Job drawing, mm, ordinate dimensions from the low corner. One solid piece. A direction names the side the tool comes from. Give positions to 0.01 mm unless a question says otherwise; leave off trailing zeros. Order: outer loops, then holes, each group sorted by start corner. A loop starts at its lowest first (then second) coordinate and runs counter-clockwise, first axis right, second up. Notation, with made-up numbers: (67, -21) - (95, -21) arc R17 cw to (95, 3) - close; hole circle Ø7 at (-26.75, 48). An arc over 180 degrees is marked (long way). Write each question's results on one line, items separated by ' | '. Start each with the question number.
1) Cut at A-A on x = 5. List the corners of the cut face in (y, z), plus the area to 3 significant figures.
2) Cut at D-D on y = 38. List the corners of the cut face in (x, z), plus the area to 3 significant figures.
3) Drill centre lines: line 1 along X through (y, z) = (4, 5) (1 decimal); line 2 along Y through (x, z) = (35, 0.9); line 3 along Y through (x, z) = (11, 6). Where is each one in solid material? Low to high. Write a range as from..to.
4) Two-plate mould, pull along X, no slides. Class the marked faces 1, 2 and 3: +X half, -X half, draft (parallel to the pull), parting line (faces both ways), or undercut.
5) Drop flat-ended pins along their axis: pin 1 Ø2 at (x, z) = (59, 4) entering from -Y; pin 2 Ø1 at (y, z) = (19, 1.5) entering from +X; pin 3 Ø4.5 at (x, z) = (5, 4) entering from -Y; pin 4 Ø15 at (x, y) = (29, 14) entering from +Z. Give the stop position or say it passes through.
6) Cut at B-B on y = 24. List the corners of the cut face in (x, z), plus the area to 3 significant figures.
7) Tool access for the marked faces 4, 5, 6, 7 and 8: list every direction of +Z, -Z, +X, -X, +Y, -Y with a clear straight run to the whole face (end or side of a thin tool).
8) Cut at C-C on z = 4. State how many separate pieces and enclosed holes the cut face has, plus the area to 3 significant figures.
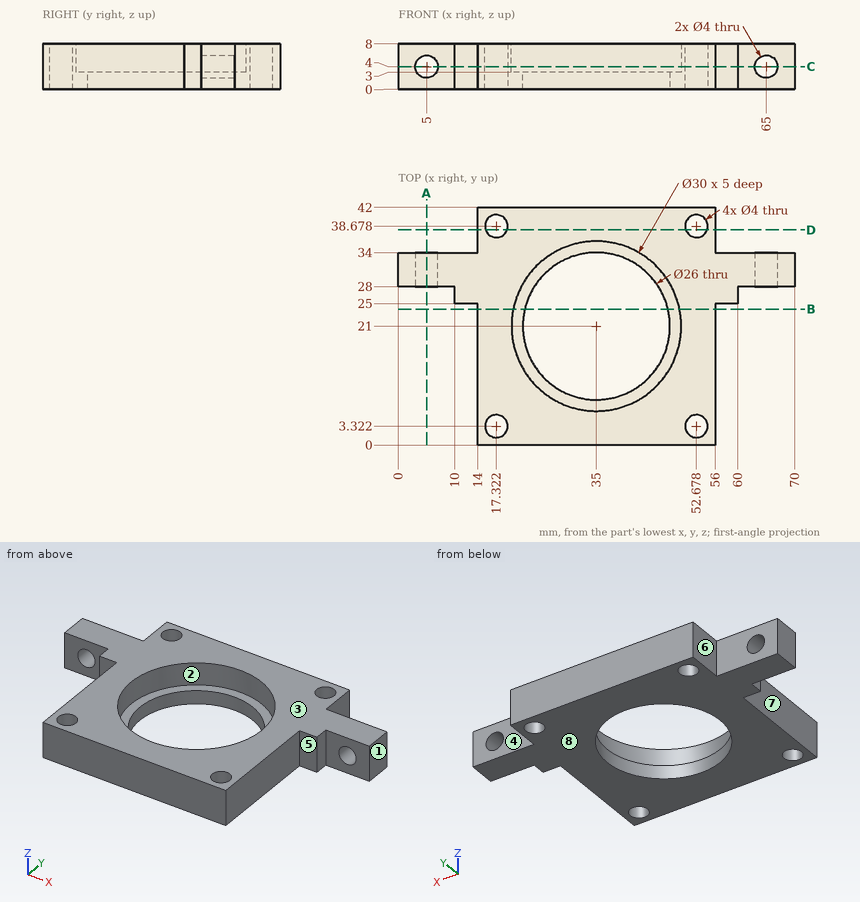
Results:
1) outline: (28, 0) - (34, 0) - (34, 2) - (28, 2) - close; (28, 6) - (34, 6) - (34, 8) - (28, 8) - close | area: 24.0 mm^2
2) outline: (14, 0) - (15.44, 0) - (15.44, 8) - (14, 8) - close; (19.2, 0) - (50.8, 0) - (50.8, 8) - (19.2, 8) - close; (54.56, 0) - (56, 0) - (56, 8) - (54.56, 8) - close | area: 276 mm^2
3) line 1: 14..15.4, 19.2..50.8, 54.6..56 | line 2: 0..8, 34..42 | line 3: 25..34
4) face 1: +X half | face 2: undercut | face 3: draft
5) pin 1: y = 25 | pin 2: x = 56 | pin 3: y = 28 | pin 4: z = 8
6) outline: (14, 0) - (22.35, 0) - (22.35, 3) - (20.3, 3) - (20.3, 8) - (14, 8) - close; (47.65, 0) - (56, 0) - (56, 8) - (49.7, 8) - (49.7, 3) - (47.65, 3) - close | area: 113 mm^2
7) face 4: +Z, -Z, +X, +Y | face 5: +Z, -Z, +X, -Y | face 6: +Z, -Z, -X, +Y | face 7: +Z, -Z, -X, -Y | face 8: -Z, +X, -X, +Y, -Y
8) separate pieces: 3 | enclosed holes: 5 | area: 1,150 mm^2
